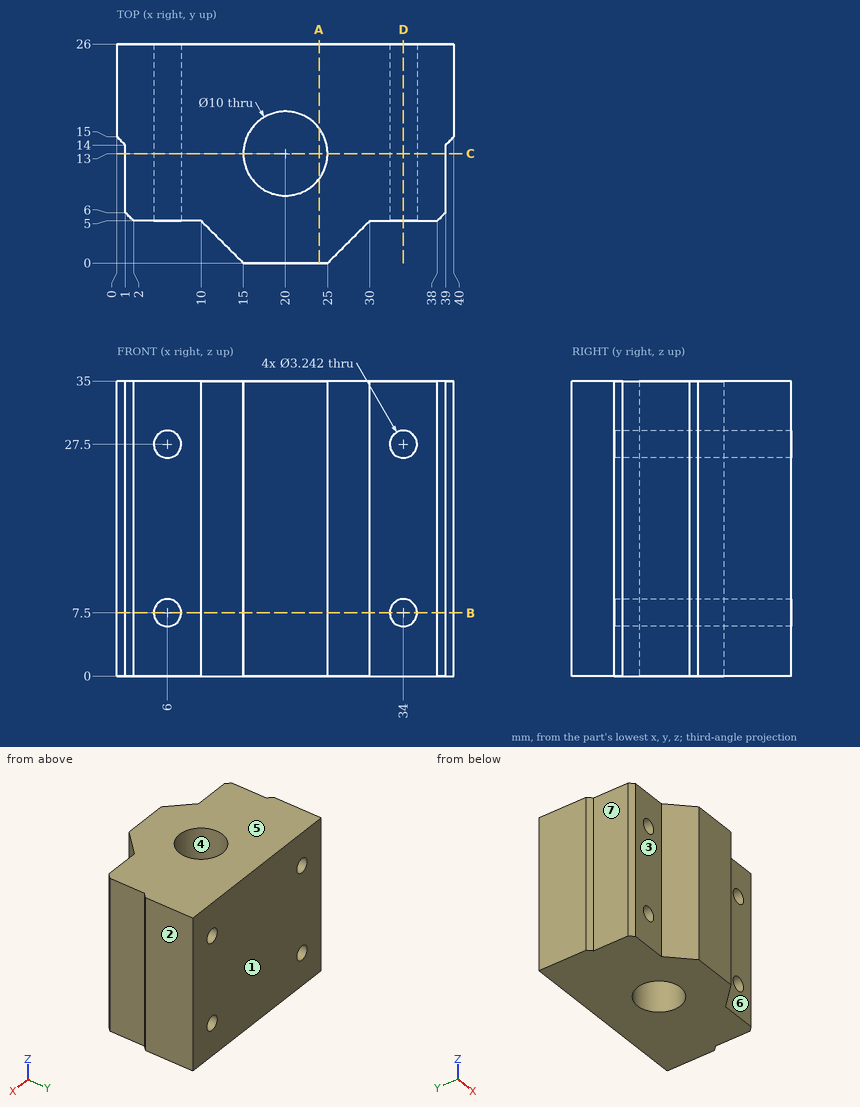
Design review of the part shown in the three views and the two pictorial views. Dimensions are in mm from the part's minimum x, y and z. A direction names the side the tool comes from. Round coordinates to 2 decimals unless told otherwise and drop trailing zeros. Loops run counter-clockwise (first coordinate to the right, second up) from the corner with the lowest first, then second, coordinate; pieces in that order, holes last. Notation, with made-up numbers: (1.5, 20.5) - (32.5, 20.5) arc R26 ccw to (32.5, 35.5) - close; hole circle Ø5 at (58, 89.5). An arc over 180 degrees is marked (long way). Write each question's results on one line, items separated by ' | '. Start each with the question number.
Q1. Wall thickness on line 1 along Z through (x, y) = (6, 18); line 2 along X through (y, z) = (6.75, 27.5); line 3 along X through (y, z) = (12.75, 27.5): over which ranges is each line inside the solid? List them lowest first. Write a range as [from, to].
Q2. Take a section at D-D on x = 34. Give the boundary of the cut face in (y, z), plus the area to 3 significant figures.
Q3. Insertion check: P1, Ø1.9, axis at x = 34, z = 7.5, coming from the -Y side; P2, Ø4, axis at x = 35.5, z = 20, coming from the -Y side; P3, Ø1.5, axis at x = 32, y = 15, coming from the -Z side; P4, Ø10, axis at x = 32.5, z = 19, coming from the -Y side. Each pin has a flat end and moves straight along its axis. Give the tip position at first contact, or say it passes through.
Q4. Take a section at C-C on y = 13. Give the boundary of the cut face in (x, z), plus the area to 3 significant figures.
Q5. Take a section at B-B on z = 7.5. Give the boundary of the cut face in (x, y).
Q6. Draft analysis for pull direction Y (two halves, no side actions). For the marked faces 1, 2, 3 and 4, state which applies: pulls with the +Y half, pulls with the -Y half, needs draft (parallel to the pull), parting line crosses it, or undercut.
Q7. Tool access review of the marked faces 5, 6 and 7: name each direction out of +Z, -Z, +X, -X, +Y, -Y from which nothing blocks a thin tool from reaching the whole face with its end or side.
Q8. Take a section at A-A on x = 24. Give the boundary of the cut face in (y, z), plus the area to 3 significant figures.
Data:
1) line 1: z = [0, 5.88], [9.12, 25.88], [29.12, 35] | line 2: x = [1, 4.38], [7.62, 32.38], [35.62, 39] | line 3: x = [1, 4.38], [7.62, 15.01], [24.99, 32.38], [35.62, 39]
2) outline: (5, 0) - (26, 0) - (26, 5.88) - (5, 5.88) - close; (5, 9.12) - (26, 9.12) - (26, 25.88) - (5, 25.88) - close; (5, 29.12) - (26, 29.12) - (26, 35) - (5, 35) - close | area: 599 mm²
3) P1: passes through | P2: stops at y = 5 | P3: stops at z = 0 | P4: stops at y = 2.5
4) outline: (1, 0) - (15, 0) - (15, 35) - (1, 35) - close; (25, 0) - (39, 0) - (39, 35) - (25, 35) - close; hole circle Ø3.24 at (6, 7.5); hole circle Ø3.24 at (6, 27.5); hole circle Ø3.24 at (34, 7.5); hole circle Ø3.24 at (34, 27.5) | area: 947 mm²
5) outline: (0, 15) - (1, 14) - (1, 6) - (2, 5) - (4.38, 5) - (4.38, 26) - (0, 26) - close; (7.62, 5) - (10, 5) - (15, 0) - (25, 0) - (30, 5) - (32.38, 5) - (32.38, 26) - (7.62, 26) - close; (35.62, 5) - (38, 5) - (39, 6) - (39, 14) - (40, 15) - (40, 26) - (35.62, 26) - close; hole circle Ø10 at (20, 13)
6) face 1: pulls with the +Y half | face 2: needs draft | face 3: pulls with the -Y half | face 4: undercut
7) face 5: +Z, +X, -X, +Y, -Y | face 6: +Z, -Z, +X, -Y | face 7: +Z, -Z, -X, -Y
8) outline: (0, 0) - (10, 0) - (10, 35) - (0, 35) - close; (16, 0) - (26, 0) - (26, 35) - (16, 35) - close | area: 700 mm²
